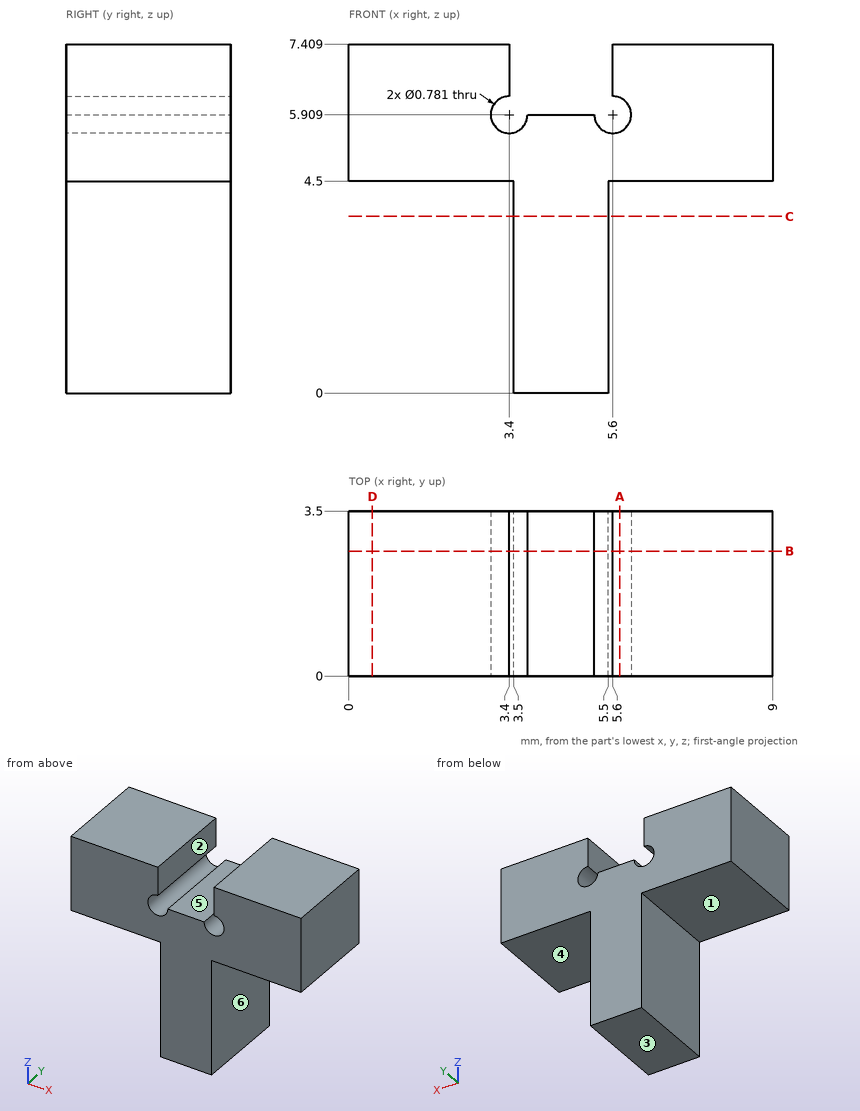
Could you check a few things on this drawing? It's one solid part, dimensions in mm from its lowest x, y, z. A direction names the side the tool comes from. Give positions to 0.01 mm unless a question says otherwise; leave off trailing zeros. Order: outer loops, then holes, each group sorted by start corner. A loop starts at its lowest first (then second) coordinate and runs counter-clockwise, first axis right, second up. Notation, with made-up numbers: (-3, -37) - (12, -37) arc R4 cw to (12, -31) - close; hole circle Ø8 at (-14.5, -21.75). An arc over 180 degrees is marked (long way). Return JSON: item names as keys, results as strings. Group by question number.
Q1. Suppose I cut it at C-C, the plane z = 3.75. Please give me the cut outline in (x, y).
Q2. Suppose I cut it at A-A, the plane x = 5.75. Please give me the cut outline in (y, z).
Q3. Thinking about a two-plate mould opening in X: for the marked faces 4, 5 and 6, which applies, pulls with the +X half, pulls with the -X half, needs draft (parallel to the pull), parting line crosses it, or undercut?
Q4. Will these pins go through, and if not, where does the flat tip stop? pin 1 Ø1.5 at (x, z) = (1, 1) entering from +Y; pin 2 Ø1 at (y, z) = (1.5, 2.5) entering from +X.
Q5. Suppose I cut it at B-B, the plane y = 2.65. Please give me the cut outline in (x, z).
Q6. Which directions (+Z, -Z, +X, -X, +Y, -Y) give clear straight access to the entire face, cutting with the end or side of a thin tool? Please do the marked faces 1, 2 and 3.
Q7. Suppose I cut it at D-D, the plane x = 0.5. Please give me the cut outline in (y, z).
Q8. Please list where these lines run through material, in increasing order: line 1 along X through (y, z) = (1.65, 7); line 2 along X through (y, z) = (1.45, 5.75); line 3 along X through (y, z) = (0.8, 6). Write a range as [from, to].
Resolved:
{
 "1": {"outline": "(3.5, 0) - (5.5, 0) - (5.5, 3.5) - (3.5, 3.5) - close"},
 "2": {"outline": "(0, 4.5) - (3.5, 4.5) - (3.5, 5.55) - (0, 5.55) - close; (0, 6.27) - (3.5, 6.27) - (3.5, 7.41) - (0, 7.41) - close"},
 "3": {"face 4": "needs draft", "face 5": "undercut", "face 6": "pulls with the +X half"},
 "4": {"pin 1": "passes through", "pin 2": "stops at x = 5.5"},
 "5": {"outline": "(0, 4.5) - (3.5, 4.5) - (3.5, 0) - (5.5, 0) - (5.5, 4.5) - (9, 4.5) - (9, 7.41) - (5.6, 7.41) - (5.6, 6.3) arc R0.39 cw (long way) to (5.21, 5.91) - (3.79, 5.91) arc R0.39 cw (long way) to (3.4, 6.3) - (3.4, 7.41) - (0, 7.41) - close"},
 "6": {"face 1": "-Z, -X, +Y, -Y", "face 2": "+Z, +Y, -Y", "face 3": "-Z, +X, -X, +Y, -Y"},
 "7": {"outline": "(0, 4.5) - (3.5, 4.5) - (3.5, 7.41) - (0, 7.41) - close"},
 "8": {"line 1": "x = [0, 3.4], [5.6, 9]", "line 2": "x = [0, 3.04], [3.76, 5.24], [5.96, 9]", "line 3": "x = [0, 3.02], [5.98, 9]"}
}
